Design review of the part built by this model. Coordinates are the model's own, in mm. Face numbers are marked on the shaded views. A direction names the side the tool comes from. Give positions to 0.01 mm unless a question says otherwise; leave off trailing zeros. Loops run counter-clockwise (first coordinate to the right, second up) from the corner with the lowest first, then second, coordinate; pieces in that order, holes last. Notation, with made-up numbers: M 70,-19 L 108,-19 A20 ccw 108,6 Z; hole C -17,37.25 d8. An arc over 180 degrees is marked long. Answer as CSV lines item,"result".
```python
from build123d import *

# Parameters (mm, degrees)
ESBO_O1_W                = 24.5
ESBO_O1_H                = 48
ESBO_O1_W_2              = 18.5
ESBO_O1_H_2              = 44.5
RESSALTO_EXTRUS_O1_DEPTH = 1
ESBO_O2_R                = 1.65
ESBO_O2_W                = 22.5
ESBO_O2_H                = 44.5
RESSALTO_EXTRUS_O2_DEPTH = 7
RESSALTO_EXTRUS_O3_DEPTH = 14.5
FILETE1_R                = 5
CHANFRO4_SIZE            = 5


with BuildPart() as part:
    # Esboço1 → Ressalto-extrusão1 (new body)
    with BuildSketch(Plane.XY):
        Rectangle(ESBO_O1_W, ESBO_O1_H)
        Rectangle(ESBO_O1_W_2, ESBO_O1_H_2, mode=Mode.SUBTRACT)
    extrude(amount=RESSALTO_EXTRUS_O1_DEPTH)

    # Esboço2 → Ressalto-extrusão2 (add)
    with BuildSketch(Plane.XY.offset(1)):
        with BuildLine():
            Line((19.25, 16), (14.25, 16))
            Line((14.25, 16), (14.25, -16))
            Line((14.25, -16), (19.25, -16))
            ThreePointArc((19.25, -16), (23.25, -20), (19.25, -24))
            Line((19.25, -24), (12.25, -24))
            Line((12.25, -24), (-12.25, -24))
            Line((-12.25, -24), (-12.25, 24))
            Line((-12.25, 24), (12.25, 24))
            Line((12.25, 24), (19.25, 24))
            ThreePointArc((19.25, 24), (23.25, 20), (19.25, 16))
        make_face()
        with Locations((19.25, 20)):
            Circle(ESBO_O2_R, mode=Mode.SUBTRACT)
        with Locations((19.25, -20)):
            Circle(ESBO_O2_R, mode=Mode.SUBTRACT)
        Rectangle(ESBO_O2_W, ESBO_O2_H, mode=Mode.SUBTRACT)
    extrude(amount=-RESSALTO_EXTRUS_O2_DEPTH)

    # Esboço4 → Ressalto-extrusão3 (add)
    with BuildSketch(Plane.XY.offset(1)):
        Polygon((-12.25, -8), (-12.25, 24), (-22.25, 18), (-22.25, 7), (-17.25, 2), (-17.25, -8), align=None)
        with BuildLine():
            ThreePointArc((-16.75, 10.8), (-18.45, 12.5), (-16.75, 14.2))
            Line((-16.75, 14.2), (-14.75, 14.2))
            ThreePointArc((-14.75, 14.2), (-13.05, 12.5), (-14.75, 10.8))
            Line((-14.75, 10.8), (-16.75, 10.8))
        make_face(mode=Mode.SUBTRACT)
    extrude(amount=-RESSALTO_EXTRUS_O3_DEPTH)

    # Filete1
    filete1_edges = [part.edges().sort_by_distance(p)[0] for p in [
        (-17.25, 2, -6.25),
        (-22.25, 7, -6.25),
        (-22.25, 18, -6.25),
    ]]
    fillet(filete1_edges, radius=FILETE1_R)

    # Chanfro4
    chanfro4_edges = [part.edges().sort_by_distance(p)[0] for p in [
        (-12.25, -8, -2.5),
    ]]
    chamfer(chanfro4_edges, length=CHANFRO4_SIZE - 0.0001)  # a hair under: the kernel refuses the full size


solid = part.part
```
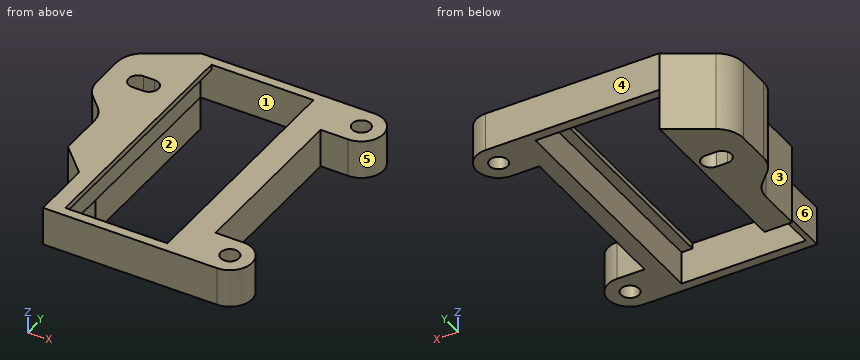
1. For P1, Ø5, axis at x = 5, y = 16.5, coming from the +Z side; P2, Ø2.5, axis at x = -15.5, z = -9.5, coming from the -Y side; P3, Ø2, axis at x = -10, y = 5, coming from the -Z side; P4, Ø6.5, axis at y = -8, z = -3.5, coming from the +X side, all flat-tipped, find the tip position at first contact; note any pin that passes through.
Answer block:
P1,"through"
P2,"y = -8"
P3,"z = 0"
P4,"x = 14.25"
2. We need section D-D, the plane z = -4. Count the separate pieces of the cut face and the enclosed holes in it, plus the area to 3 significant figures.
Answer block:
separate pieces,"1"
enclosed holes,"4"
area,"607 mm²"
3. The part is to be moulded in two halves that separate along Y. For the marked faces 4, 5 and 6, say which applies: pulls with the +Y half, pulls with the -Y half, needs draft (parallel to the pull), parting line crosses it, or undercut.
Answer block:
face 4,"pulls with the +Y half"
face 5,"undercut"
face 6,"needs draft"
4. To check wall thickness, follow L1, parallel to Y at x = 19.25, z = -1; L2, parallel to Y at x = 6.5, z = -0.5; L3, parallel to X at y = 0, z = -0.5. State the ranges of each line that lie inside material, in increasing order. Write a range as [from, to].
Answer block:
L1,"[-24, -21.65], [-18.35, -16], [16, 18.35], [21.65, 24]"
L2,"[-24, -22.25], [22.25, 24]"
L3,"[-17.25, -11.25], [11.25, 14.25]"
5. For the marked faces 1, 2 and 3, list the 3-axis set-ups (+Z, -Z, +X, -X, +Y, -Y) from which the entire face can be reached by the end or side of a thin tool; tool diameter is ignored.
Answer block:
face 1,"-Z"
face 2,"-Z, +X, +Y, -Y"
face 3,"+Z, -Z, -X, -Y"
6. We need section B-B, the plane y = 12.5. Write out the cut boundary in (x, z), plus the area to 3 significant figures.
Answer block:
outline,"M -22.25,-13.5 L -18.45,-13.5 L -18.45,1 L -22.25,1 Z; M -13.05,-13.5 L -12.25,-13.5 L -12.25,-6 L -11.25,-6 L -11.25,0 L -9.25,0 L -9.25,1 L -13.05,1 Z; M 9.25,0 L 11.25,0 L 11.25,-6 L 14.25,-6 L 14.25,1 L 9.25,1 Z"
area,"98.7 mm²"
7. We need section C-C, the plane z = -9.5. Write out the cut boundary in (x, y).
Answer block:
outline,"M -22.25,9.07 A5 ccw -20.79,5.54 L -18.71,3.46 A5 cw -17.25,-0.07 L -17.25,-8 L -12.25,-8 L -12.25,24 L -19.82,19.46 A5 ccw -22.25,15.17 Z; hole M -16.75,10.8 L -14.75,10.8 A1.7 ccw -14.75,14.2 L -16.75,14.2 A1.7 ccw Z"
8. We need section A-A, the plane x = -5.5. Write out the cut boundary in (y, z).
Answer block:
outline,"M -24,-6 L -22.25,-6 L -22.25,1 L -24,1 Z; M 22.25,-6 L 24,-6 L 24,1 L 22.25,1 Z"
